```python
from build123d import *

# Parameters (mm, degrees)
SKETCH_1_R      = 19.32
EXTRUDE_1_DEPTH = 42
SKETCH_2_W      = 15.375163756
SKETCH_2_H      = 36.857684224
EXTRUDE_2_DEPTH = 42


with BuildPart() as part:
    # Эскиз1 → Бобышка-Вытянуть1 (new body)
    with BuildSketch(Plane(origin=(0, 0, 0), x_dir=(1, 0, 0), z_dir=(0, 1, 0))):
        Circle(SKETCH_1_R)
    extrude(amount=EXTRUDE_1_DEPTH)

    # Эскиз2 → Бобышка-Вытянуть2 (add)
    with BuildSketch(Plane.XZ):
        Rectangle(SKETCH_2_W, SKETCH_2_H)
    extrude(amount=EXTRUDE_2_DEPTH)


solid = part.part
```
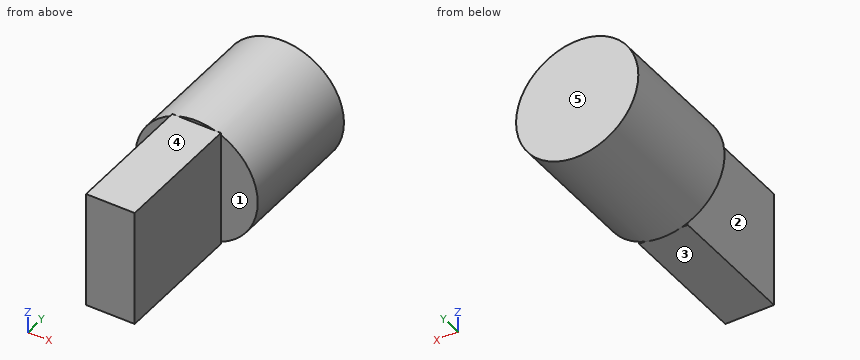
Read the model definition and answer for the solid it produces. Units are mm, in the model's axes. Face numbers are marked on the shaded views. A direction names the side the tool comes from. Give positions to 0.01 mm unless a question says otherwise; leave off trailing zeros. Order: outer loops, then holes, each group sorted by start corner. A loop starts at its lowest first (then second) coordinate and runs counter-clockwise, first axis right, second up.
(1) Find section B-B (x = 0). Give the vertices of the cut face in (y, z), plus the area to 3 significant figures.
(2) Straight lines are drawn through the part: L1, parallel to X at y = -32.5, z = -5; L2, parallel to Z at x = 4.5, y = -15.5; L3, parallel to Y at x = 15.5, z = 0. For each, find the intervals that lie inside material, in ascending order.
(3) For the marked faces 1, 2, 3, 4 and 5, determine the directions among +Z, -Z, +X, -X, +Y, -Y from which every point of the face is accessible in a straight line to the end or side of a thin tool.
(4) Find section D-D (y = 18.5). Give the vertices of the cut face in (x, z), plus the area to 3 significant figures.
(5) Given pin 1 (18.5 mm diameter, centred on y = -18, z = 0, fed in from +X); pin 2 (1 mm diameter, centred on x = -2.5, z = 19, fed in from -Y); pin 3 (8 mm diameter, centred on x = -5, y = -30.5, fed in from +Z), each flat-ended and moving along its own axis, determine where each tip first touches the part or whether it passes through.
(6) Find section C-C (y = -10). Give the vertices of the cut face in (x, z).
(7) Find section A-A (z = 0). Give the vertices of the cut face in (x, y), plus the area to 3 significant figures.
Result sheet:
1. outline: (-42, -18.43) - (0, -18.43) - (0, -19.32) - (42, -19.32) - (42, 19.32) - (0, 19.32) - (0, 18.43) - (-42, 18.43) - close
1. area: 3,170 mm2
2. L1: x = -7.69 to 7.69
2. L2: z = -18.43 to 18.43
2. L3: y = 0 to 42
3. face 1: +Z, -Z, +X, -Y
3. face 2: +Z, -Z, -X, -Y
3. face 3: -Z, +X, -X, -Y
3. face 4: +Z, +X, -X, -Y
3. face 5: +Z, -Z, +X, -X, +Y
4. outline: circle Ø38.64 at (0, 0)
4. area: 1,170 mm2
5. pin 1: stops at x = 7.69
5. pin 2: stops at y = 0
5. pin 3: stops at z = 18.43
6. outline: (-7.69, -18.43) - (7.69, -18.43) - (7.69, 18.43) - (-7.69, 18.43) - close
7. outline: (-19.32, 0) - (-7.69, 0) - (-7.69, -42) - (7.69, -42) - (7.69, 0) - (19.32, 0) - (19.32, 42) - (-19.32, 42) - close
7. area: 2,270 mm2
